Autodesk Inventor part; units mm, degrees
ref_plane "YZ Plane" through (0, 0, 0) normal (1, 0, 0) x (0, 1, 0)
ref_plane "XZ Plane" through (0, 0, 0) normal (0, 1, 0) x (-1, 0, 0)
ref_plane "XY Plane" through (0, 0, 0) normal (0, 0, 1) x (1, 0, 0)
sketch "Sketch1" plane through (0, 0, 0) normal (0, 0, 1) x (1, 0, 0)
  line L0 (0, 0) -> (25.4, 0)
  line L1 (25.4, 0) -> (25.4, 25.4)
  line L2 (25.4, 25.4) -> (0, 25.4)
  line L3 (0, 25.4) -> (0, 0)
  dimension "d0" = 25.4
  dimension "d1" = 25.4
extrude "Extrusion1" add sketch "Sketch1" along normal blind 863.6
fillet "Fillet1" radius 12.7 4 edges at (12.7, 25.4, 863.6) (12.7, 0, 863.6) (12.7, 25.4, 0) (12.7, 0, 0)
sketch "Sketch2" plane through (0, 0, 0) normal (0, 0, 1) x (1, 0, 0)
  line L0 (22.86, 22.86) -> (2.54, 22.86)
  line L1 (2.54, 22.86) -> (2.54, 2.54)
  line L2 (2.54, 2.54) -> (22.86, 2.54)
  line L3 (22.86, 2.54) -> (22.86, 22.86)
  line L4 (0, 25.4) -> (25.4, 25.4)
  line L5 (0, 0) -> (0, 25.4)
  line L6 (25.4, 0) -> (0, 0)
  line L7 (25.4, 25.4) -> (25.4, 0)
  dimension "d5" = 2.54
  dimension "d6" = 2.54
  dimension "d7" = 2.54
  dimension "d8" = 2.54
extrude "Extrusion2" cut sketch "Sketch2" along normal blind 1016 contours L3 L2 L1 L0
sketch "Sketch3" plane through (0, 12.7, 12.7) normal (-1, 0, 0) x (0, 0, 1)
  circle A0 centre (0, 0) radius 7.8422
  circle A1 centre (27.94, 0) radius 7.8422
  circle A2 centre (55.88, 0) radius 7.8422
  circle A3 centre (83.82, 0) radius 7.8423
  circle A4 centre (838.2, 0) radius 7.8423
  circle A5 centre (810.26, 0) radius 7.8422
  circle A6 centre (782.32, 0) radius 7.8422
  circle A7 centre (754.38, 0) radius 7.8423
  line L0 (0, 12.7) -> (838.2, 12.7)
  arc A8 (0, 12.7) -> (0, -12.7) centre (0, 0) ccw
  arc A9 (838.2, -12.7) -> (838.2, 12.7) centre (838.2, 0) ccw
  point P0 (-12.7, -12.7)
  dimension "d11" = 15.6845
  dimension "d12" = 15.6845
  dimension "d13" = 15.6845
  dimension "d14" = 15.6845
  dimension "d15" = 15.6845
  dimension "d16" = 15.6845
  dimension "d17" = 15.6845
  dimension "d18" = 15.6845
  dimension "d19" = 12.7
  dimension "d20" = 12.7
  dimension "d21" = 12.7
  dimension "d22" = 12.7
  dimension "d23" = 12.7
  dimension "d24" = 12.7
  dimension "d25" = 12.7
  dimension "d26" = 12.7
  dimension "d27" = 0
  dimension "d28" = 27.94
  dimension "d29" = 27.94
  dimension "d30" = 27.94
  dimension "d31" = 0
  dimension "d32" = 27.94
  dimension "d33" = 27.94
  dimension "d34" = 27.94
extrude "Extrusion3" cut sketch "Sketch3" against normal blind 25.4
equation "\"d29\" = d28"
equation "\"d30\" = d28"
equation "\"d33\" = d32"
equation "\"d34\" = d32"
properties part number "Support Pivs 25 uppermiddle"
Here's how the part is built. I have some questions about the finished solid (model axes, mm). A direction names the side the tool comes from. Round coordinates to 2 decimals unless told otherwise and drop trailing zeros. Order: outer loops, then holes, each group sorted by start corner. A loop starts at its lowest first (then second) coordinate and runs counter-clockwise, first axis right, second up. Notation, with made-up numbers: M 84,-18 L 107,-18 A32 ccw 107,12 Z; hole C -32,26 d2. An arc over 180 degrees is marked long. Return JSON: item names as keys, results as strings. Group by question number.
1. If we section it at A-A on z = 767.08: List the corners of the cut face in (x, y) for me.
2. If we mould it in two halves opening along Z, with no side actions, what happens to faces 1 (the face through (2.54, 13, 426)), 2 (the face through (1.252, 5.044, 38.94)), 3 (the face through (1.252, 9.696, 75.824))? For each: pulls with the +Z half, pulls with the -Z half, needs draft (parallel to the pull), parting line crosses it, or undercut.
3. If we section it at B-B on x = 8.25: List the corners of the cut face in (y, z) for me.
4. Please list where these lines run through material, in increasing order: probe 1 along Y at (x, z) = (8.5, 651); probe 2 along Y at (x, z) = (1.95, 767.08).
5. If we section it at C-C on z = 310: List the corners of the cut face in (x, y) for me.
6. On a 3-axis mill with a long thin cutter (end or side, diameter ignored), from which of +Z, -Z, +X, -X, +Y, -Y can I reach the whole of each face in a straight line? I mean faces 4 (the face through (1.25, 15.06, 774.56)), 5 (the face through (13, 2.54, 426)). Say none if no direction works.
7. I'm going to push flat-ended pins straight in: pin 1 Ø9.5 at (y, z) = (12.7, 96.52) entering from +X; pin 2 Ø3 at (x, y) = (6.5, 21.5) entering from -Z; pin 3 Ø5 at (x, y) = (3.5, 7.5) entering from -Z. Where does each tip first touch, or does it pass through?
Reply:
{
 "1": {"outline": "M 0,0 L 25.4,0 L 25.4,4.86 L 22.86,4.86 L 22.86,2.54 L 2.54,2.54 L 2.54,4.86 L 0,4.86 Z; M 0,20.54 L 2.54,20.54 L 2.54,22.86 L 22.86,22.86 L 22.86,20.54 L 25.4,20.54 L 25.4,25.4 L 0,25.4 Z"},
 "2": {"face 1": "needs draft", "face 2": "undercut", "face 3": "undercut"},
 "3": {"outline": "M 0,12.7 A12.7 ccw 2.54,5.08 L 2.54,858.52 A12.7 ccw 0,850.9 Z; M 22.86,5.08 A12.7 ccw 25.4,12.7 L 25.4,850.9 A12.7 ccw 22.86,858.52 Z"},
 "4": {"probe 1": "0 to 2.54, 22.86 to 25.4", "probe 2": "0 to 4.86, 20.54 to 25.4"},
 "5": {"outline": "M 0,0 L 25.4,0 L 25.4,25.4 L 0,25.4 Z; hole M 2.54,2.54 L 22.86,2.54 L 22.86,22.86 L 2.54,22.86 Z"},
 "6": {"face 4": "+X, -X", "face 5": "+Z, -Z"},
 "7": {"pin 1": "through", "pin 2": "z = 5.08", "pin 3": "z = 0.33"}
}
